The drawing under review shows one solid part. Ordinate dimensions are in mm from its lowest x, y, z. Give positions to 0.01 mm unless a question says otherwise; leave off trailing zeros. Loops run counter-clockwise (first coordinate to the right, second up) from the corner with the lowest first, then second, coordinate; pieces in that order, holes last. Notation, with made-up numbers: (75, -7) - (93, -7) arc R25 ccw to (93, 21) - close; hole circle Ø1 at (70, 12.25). An arc over 180 degrees is marked (long way). Write each question's results on one line, items separated by ' | '.
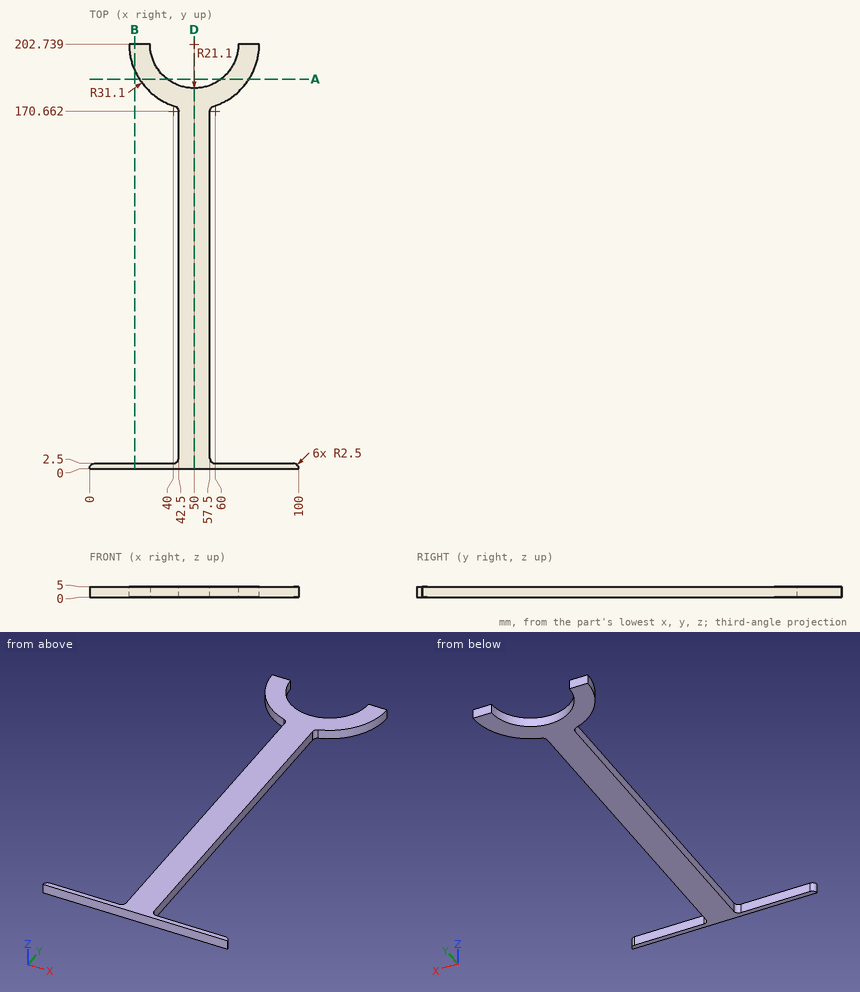
(1) Take a section at B-B on x = 21.5. Give the boundary of the cut face in (y, z).
Answers below:
outline: (0, 0) - (2.5, 0) - (2.5, 5) - (0, 5) - close; (190.29, 0) - (202.74, 0) - (202.74, 5) - (190.29, 5) - close
(2) Take a section at A-A on y = 186. Give the boundary of the cut face in (x, z), plus the area to 3 significant figures.
Answers below:
outline: (23.79, 0) - (37.15, 0) - (37.15, 5) - (23.79, 5) - close; (62.85, 0) - (76.21, 0) - (76.21, 5) - (62.85, 5) - close | area: 134 mm2
(3) Take a section at D-D on x = 50. Give the boundary of the cut face in (y, z), plus the area to 3 significant figures.
Answers below:
outline: (0, 0) - (181.64, 0) - (181.64, 5) - (0, 5) - close | area: 908 mm2
(4) Insertion check: P1, Ø2, axis at y = 154, z = 3, coming from the -X side; P2, Ø1.5, axis at y = 125.5, z = 2, coming from the +X side; P3, Ø2.5, axis at x = 86, z = 3, coming from the +Y side. Each pin has a flat end and moves straight along its axis. Give the tip position at first contact, or say it passes through.
Answers below:
P1: x = 42.5 | P2: x = 57.5 | P3: y = 2.5
(5) Wall thickness on line 1 along X through (y, z) = (20.5, 4.4); line 2 along Y through (x, z) = (38.5, 2.9); line 3 along Y through (x, z) = (34.5, 1.15): over which ranges is each line inside the solid? List them lowest first. Write a range as from..to.
Answers below:
line 1: 42.5..57.5 | line 2: 0..2.5, 173.84..185.05 | line 3: 0..2.5, 175.78..188.42
